The model under review builds one solid part; all positions refer to its coordinate system, in mm. Face numbers are marked on the shaded views. A direction names the side the tool comes from. Coordinates: 2 decimals unless noted, no trailing zeros. Write each loop counter-clockwise with the first axis right and the second up, starting at its lowest first coordinate (ties: lowest second). Pieces come first, ordered by that corner, then holes. Notation, with made-up numbers: (-19.75, 12.5) -> (-1.75, 12.5) arc R27 ccw to (-1.75, 45.5) -> close; hole circle Ø11 at (-2.5, -12). An arc over 180 degrees is marked (long way). Write each question's results on one line, items separated by ' | '.
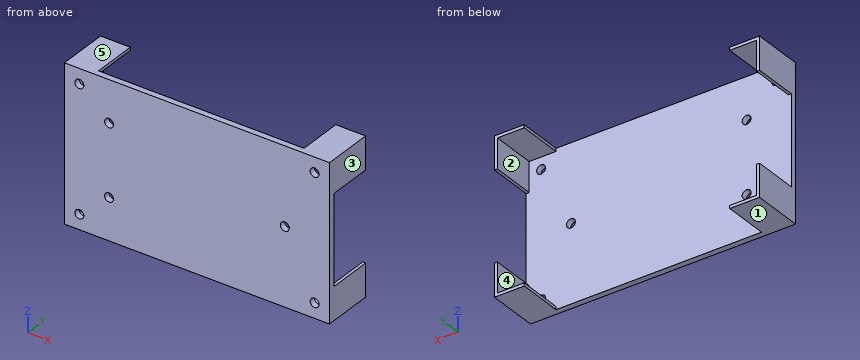
```python
from build123d import *

# Parameters (mm, degrees)
SKETCH1_W           = 89
SKETCH1_H           = 52
BOSS_EXTRUDE1_DEPTH = 2
SKETCH2_R           = 1.5
CUT_EXTRUDE1_DEPTH  = 3
SKETCH5_R           = 1.5
CUT_EXTRUDE3_DEPTH  = 3
BOSS_EXTRUDE3_DEPTH = 15


with BuildPart() as part:
    # Sketch1 → Boss-Extrude1 (new body)
    with BuildSketch(Plane(origin=(0, 0, 0), x_dir=(1, 0, 0), z_dir=(0, 1, 0))):
        with Locations((-15.729105331, -13.267137121)):
            Rectangle(SKETCH1_W, SKETCH1_H)
    extrude(amount=BOSS_EXTRUDE1_DEPTH)

    # Sketch2 → Cut-Extrude1 (cut, through all)
    with BuildSketch(Plane(origin=(0, 2, 0), x_dir=(1, 0, 0), z_dir=(0, 1, 0))):
        with Locations((-55.229105331, -34.267137121)):
            Circle(SKETCH2_R)
        with Locations((-55.229105331, 7.732862879)):
            Circle(SKETCH2_R)
        with Locations((23.770894669, 7.732862879)):
            Circle(SKETCH2_R)
        with Locations((23.770894669, -34.267137121)):
            Circle(SKETCH2_R)
    extrude(amount=-CUT_EXTRUDE1_DEPTH, mode=Mode.SUBTRACT)

    # Sketch5 → Cut-Extrude3 (cut, through all)
    with BuildSketch(Plane(origin=(0, 2, 0), x_dir=(1, 0, 0), z_dir=(0, 1, 0))):
        with Locations((-45.229105331, -25.267137121)):
            Circle(SKETCH5_R)
        with Locations((-45.229105331, -1.267137121)):
            Circle(SKETCH5_R)
        with Locations((13.770894669, -13.267137121)):
            Circle(SKETCH5_R)
    extrude(amount=-CUT_EXTRUDE3_DEPTH, mode=Mode.SUBTRACT)

    # Sketch6 → Boss-Extrude3 (add)
    with BuildSketch(Plane(origin=(0, 2, 0), x_dir=(1, 0, 0), z_dir=(0, 1, 0))):
        Polygon((-60.229105331, -28.267137121), (-60.229105331, -39.267137121), (-50.229105331, -39.267137121), (-50.229105331, -38.267137121), (-59.229105331, -38.267137121), (-59.229105331, -28.267137121), align=None)
        Polygon((-60.229105331, 1.732862879), (-59.229105331, 1.732862879), (-59.229105331, 11.732862879), (-50.229105331, 11.732862879), (-50.229105331, 12.732862879), (-60.229105331, 12.732862879), align=None)
        Polygon((27.770894669, -28.267137121), (27.770894669, -38.267137121), (18.770894669, -38.267137121), (18.770894669, -39.267137121), (28.770894669, -39.267137121), (28.770894669, -28.267137121), align=None)
        Polygon((27.770894669, 11.732862879), (27.770894669, 1.732862879), (28.770894669, 1.732862879), (28.770894669, 12.732862879), (18.770894669, 12.732862879), (18.770894669, 11.732862879), align=None)
    extrude(amount=BOSS_EXTRUDE3_DEPTH)


solid = part.part
```
Q1. Machinability: for the marked faces 1 and 2, which of the approach directions +Z, -Z, +X, -X, +Y, -Y give a long, thin tool a straight path to every point of the face, cutting with its end or side? Answer none if there is none.
Solution:
face 1: -Z, +X, -X, +Y, -Y | face 2: +Y
Q2. Clearance check with a flat-ended pin moving along its axis: P1, Ø5, axis at x = -22.5, z = -2, coming from the +Y side. State where the tip first meets the part, or that it passes through.
Solution:
P1: y = 2
Q3. Draft analysis for pull direction Z (two halves, no side actions). For the marked faces 3, 4 and 5, state which applies: pulls with the +Z half, pulls with the -Z half, needs draft (parallel to the pull), parting line crosses it, or undercut.
Solution:
face 3: needs draft | face 4: undercut | face 5: pulls with the +Z half
Q4. Add section C-C (z = 20). Write out the cut boundary in (x, y).
Solution:
outline: (-60.23, 0) -> (28.77, 0) -> (28.77, 2) -> (-60.23, 2) -> close
Q5. For line 1 (X direction, y = 8.25, z = 37); line 2 (Y direction, x = 24, z = 13), list the stretches that pass through material, from the lowest coordinate up. Write a range as from..to.
Solution:
line 1: -60.23..-59.23, 27.77..28.77 | line 2: 0..2
Q6. Add section A-A (y = 10.5). Write out the cut boundary in (x, z), plus the area to 3 significant figures.
Solution:
outline: (-60.23, -12.73) -> (-50.23, -12.73) -> (-50.23, -11.73) -> (-59.23, -11.73) -> (-59.23, -1.73) -> (-60.23, -1.73) -> close; (-60.23, 28.27) -> (-59.23, 28.27) -> (-59.23, 38.27) -> (-50.23, 38.27) -> (-50.23, 39.27) -> (-60.23, 39.27) -> close; (18.77, -12.73) -> (28.77, -12.73) -> (28.77, -1.73) -> (27.77, -1.73) -> (27.77, -11.73) -> (18.77, -11.73) -> close; (18.77, 38.27) -> (27.77, 38.27) -> (27.77, 28.27) -> (28.77, 28.27) -> (28.77, 39.27) -> (18.77, 39.27) -> close | area: 80.0 mm²
Q7. Add section B-B (x = 5). Write out the cut boundary in (y, z), plus the area to 3 significant figures.
Solution:
outline: (0, -12.73) -> (2, -12.73) -> (2, 39.27) -> (0, 39.27) -> close | area: 104 mm²
